For this review, take the finished solid that the model builds, in its own axes (mm). Round coordinates to 2 decimals unless told otherwise and drop trailing zeros. Loops run counter-clockwise (first coordinate to the right, second up) from the corner with the lowest first, then second, coordinate; pieces in that order, holes last.
1. Consider section B-B on x = -63. State the section outline as (y, z) points.
2. To check wall thickness, follow line 1 along X through (y, z) = (4, 70); line 2 along X through (y, z) = (7.75, -15.5); line 3 along Z through (x, y) = (30, 7.25). State the ranges of each line that lie inside material, in increasing order.
3. Consider section C-C on z = -77.5. State the section outline as (x, y) points, then the cut area to 3 significant figures.
4. Clearance check with flat-ended pins moving along their axes: pin 1 Ø4.5 at (x, z) = (-13.44, 13.44) entering from +Y; pin 2 Ø5 at (x, y) = (73.5, 3) entering from +Z; pin 3 Ø6 at (y, z) = (6.5, -57.5) entering from -X. State where each tip first meets the part, or that it passes through.
5. Consider section A-A on y = 3.5. State how many separate pieces and enclosed holes the cut face has, then the cut area to 3 significant figures.
from build123d import *

# Parameters (mm, degrees)
SKETCH_1_R          = 60
EXTRUDE_1_DEPTH     = 10
SKETCH_2_R          = 1.7
SKETCH_2_R_2        = 3.925573477
CUT_EXTRUDE_1_DEPTH = 10
SKETCH_3_R          = 1.7
CUT_EXTRUDE_2_DEPTH = 10
SKETCH_4_R          = 3.7
CUT_EXTRUDE_3_DEPTH = 4.5
SKETCH_5_R          = 3.893175391
SKETCH_5_R_2        = 3.7
EXTRUDE_2_DEPTH     = 10
SKETCH_6_R          = 1.7
CUT_EXTRUDE_4_DEPTH = 10


with BuildPart() as part:
    # 草图1 → 凸台-拉伸1 (new body)
    with BuildSketch(Plane(origin=(0, 0, 0), x_dir=(1, 0, 0), z_dir=(0, 1, 0))):
        Circle(SKETCH_1_R)
    extrude(amount=EXTRUDE_1_DEPTH)

    # 草图2 → 切除-拉伸1 (cut)
    with BuildSketch(Plane(origin=(0, 10, 0), x_dir=(1, 0, 0), z_dir=(0, 1, 0))):
        with Locations((-13.435028843, 13.435028843)):
            Circle(SKETCH_2_R)
        Circle(SKETCH_2_R_2)
        with Locations((13.435028843, 13.435028843)):
            Circle(SKETCH_2_R)
        with Locations((13.435028843, -13.435028843)):
            Circle(SKETCH_2_R)
        with Locations((-13.435028843, -13.435028843)):
            Circle(SKETCH_2_R)
    extrude(amount=-CUT_EXTRUDE_1_DEPTH, mode=Mode.SUBTRACT)

    # 草图3 → 切除-拉伸2 (cut)
    with BuildSketch(Plane(origin=(0, 10, 0), x_dir=(1, 0, 0), z_dir=(0, 1, 0))):
        with Locations((-30, 40)):
            Circle(SKETCH_3_R)
        with Locations((30, 40)):
            Circle(SKETCH_3_R)
        with Locations((-30, -40)):
            Circle(SKETCH_3_R)
        with Locations((30, -40)):
            Circle(SKETCH_3_R)
    extrude(amount=-CUT_EXTRUDE_2_DEPTH, mode=Mode.SUBTRACT)

    # 草图4 → 切除-拉伸3 (cut)
    with BuildSketch(Plane(origin=(0, 10, 0), x_dir=(1, 0, 0), z_dir=(0, 1, 0))):
        with Locations((-13.435028843, 13.435028843)):
            Circle(SKETCH_4_R)
        with Locations((13.435028843, 13.435028843)):
            Circle(SKETCH_4_R)
        with Locations((13.435028843, -13.435028843)):
            Circle(SKETCH_4_R)
        with Locations((-13.435028843, -13.435028843)):
            Circle(SKETCH_4_R)
        with Locations((-30, 40)):
            Circle(SKETCH_4_R)
        with Locations((30, 40)):
            Circle(SKETCH_4_R)
        with Locations((-30, -40)):
            Circle(SKETCH_4_R)
        with Locations((30, -40)):
            Circle(SKETCH_4_R)
    extrude(amount=-CUT_EXTRUDE_3_DEPTH, mode=Mode.SUBTRACT)

    # 草图5 → 凸台-拉伸2 (add)
    with BuildSketch(Plane(origin=(0, 10, 0), x_dir=(1, 0, 0), z_dir=(0, 1, 0))):
        Polygon((25, 25), (25, 90), (-25, 90), (-25, 25), (-90, 25), (-90, -25), (-25, -25), (-25, -90), (25, -90), (25, -25), (90, -25), (90, 25), align=None)
        Circle(SKETCH_5_R, mode=Mode.SUBTRACT)
        with Locations((13.435028843, 13.435028843)):
            Circle(SKETCH_5_R_2, mode=Mode.SUBTRACT)
        with Locations((-13.435028843, 13.435028843)):
            Circle(SKETCH_5_R_2, mode=Mode.SUBTRACT)
        with Locations((-13.435028843, -13.435028843)):
            Circle(SKETCH_5_R_2, mode=Mode.SUBTRACT)
        with Locations((13.435028843, -13.435028843)):
            Circle(SKETCH_5_R_2, mode=Mode.SUBTRACT)
    extrude(amount=-EXTRUDE_2_DEPTH)

    # 草图6 → 切除-拉伸4 (cut)
    with BuildSketch(Plane.XZ):
        with Locations((0, -70)):
            Circle(SKETCH_6_R)
        with Locations((-70, 0)):
            Circle(SKETCH_6_R)
        with Locations((0, 70)):
            Circle(SKETCH_6_R)
        with Locations((70, 0)):
            Circle(SKETCH_6_R)
    extrude(amount=-CUT_EXTRUDE_4_DEPTH, mode=Mode.SUBTRACT)


solid = part.part
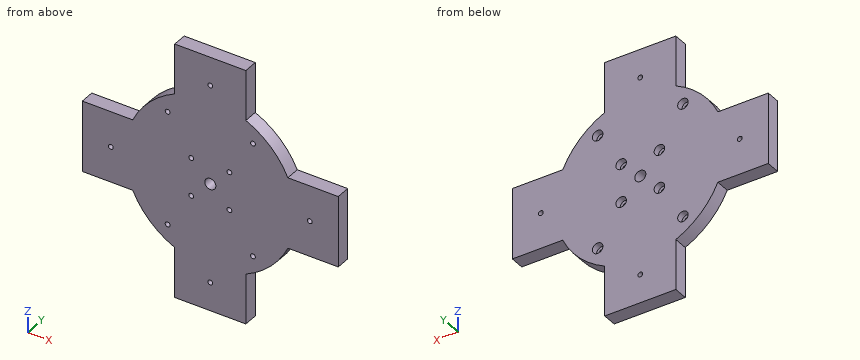
Resolved:
1. outline: (0, -25) - (10, -25) - (10, 25) - (0, 25) - close
2. line 1: x = -25 to -1.7, 1.7 to 25
2. line 2: x = -90 to -16.51, -10.36 to 10.36, 16.51 to 90
2. line 3: z = -51.96 to -43.7, -36.3 to 36.3, 43.7 to 51.96
3. outline: (-25, 0) - (25, 0) - (25, 10) - (-25, 10) - close
3. area: 500 mm2
4. pin 1: stops at y = 5.5
4. pin 2: stops at z = 25
4. pin 3: stops at x = -25.09
5. separate pieces: 1
5. enclosed holes: 13
5. area: 17,500 mm2
